Geometry: final body of the model. Coordinates: model frame, mm. Face numbers are marked on the shaded views. Round coordinates to 2 decimals unless told otherwise and drop trailing zeros. Loops run counter-clockwise (first coordinate to the right, second up) from the corner with the lowest first, then second, coordinate; pieces in that order, holes last. Notation, with made-up numbers: M 89,-19.75 L 100,-19.75 A20 ccw 100,12.25 Z; hole C -24.75,4.25 d6. An arc over 180 degrees is marked long. Write each question's results on one line, items separated by ' | '.
```python
from build123d import *

# Parameters (mm, degrees)
F0_R     = 5.5
F1_DEPTH = 13.6
F2_R     = 8.165
F3_DEPTH = 1.82
F4_R     = 5.65
F5_DEPTH = 25
F6_R     = 4.5
F7_DEPTH = 40.421
F8_R     = 1.45
F9_DEPTH = 12


with BuildPart() as f1:
    # F0 (on Top) → F1 (new body)
    with BuildSketch(Plane.XY):
        Circle(F0_R)
    extrude(amount=F1_DEPTH)

    # F2 (on face) → F3 (join)
    with BuildSketch(Plane.XY.offset(13.6)):
        Circle(F2_R)
    extrude(amount=F3_DEPTH)

    # F4 (on face) → F5 (join)
    with BuildSketch(Plane.XY.offset(15.42)):
        Circle(F4_R)
    extrude(amount=F5_DEPTH)

    # F6 (on face) → F7 (cut, through all)
    with BuildSketch(Plane(origin=(0, 0, 0), x_dir=(1, 0, 0), z_dir=(0, 0, -1))):
        Circle(F6_R)
    extrude(amount=-F7_DEPTH, mode=Mode.SUBTRACT)

    # F8 (on Front) → F9 (cut)
    with BuildSketch(Plane.XZ):
        with Locations((0, 25)):
            Circle(F8_R)
        with Locations((0, 5)):
            Circle(F8_R)
    extrude(amount=F9_DEPTH, mode=Mode.SUBTRACT)


solid = f1.part
```
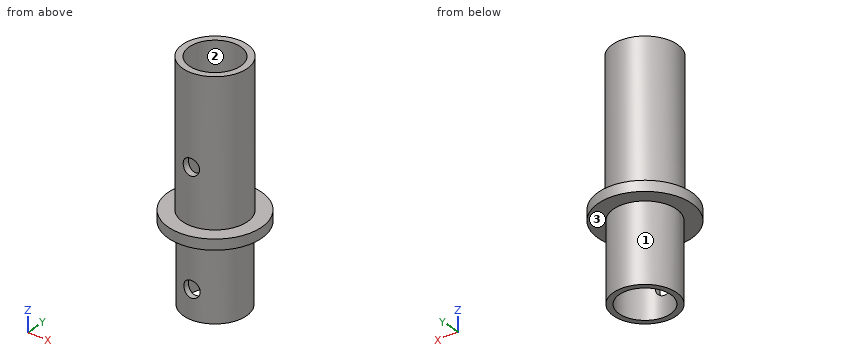
1. Pin query (flat end, axial travel): P1, Ø3, axis at x = -2.5, z = 14.5, coming from the +Y side; P2, Ø4, axis at x = 0, z = 25, coming from the -Y side; P3, Ø1.5, axis at y = -4, z = 11, coming from the +X side. Return the tip coordinate at first contact, or that it passes through.
Answer key:
P1: stops at y = 8.1 | P2: stops at y = -5.65 | P3: stops at x = 4.44
2. Section B-B (x = 0). Output: boundary loops of the cut face in (y, z) (3 decimals), then the cut area to 3 significant figures.
Answer key:
outline: M -8.165,13.6 L -5.5,13.6 L -5.5,6.45 L -4.5,6.45 L -4.5,23.55 L -5.65,23.55 L -5.65,15.42 L -8.165,15.42 Z; M -5.65,26.45 L -4.5,26.45 L -4.5,40.42 L -5.65,40.42 Z; M -5.5,0 L -4.5,0 L -4.5,3.55 L -5.5,3.55 Z; M 4.5,0 L 5.5,0 L 5.5,13.6 L 8.165,13.6 L 8.165,15.42 L 5.65,15.42 L 5.65,40.42 L 4.5,40.42 Z | area: 91.8 mm²
3. Section A-A (y = 0). Output: boundary loops of the cut face in (x, z) (3 decimals).
Answer key:
outline: M -8.165,13.6 L -5.5,13.6 L -5.5,0 L -4.5,0 L -4.5,40.42 L -5.65,40.42 L -5.65,15.42 L -8.165,15.42 Z; M 4.5,0 L 5.5,0 L 5.5,13.6 L 8.165,13.6 L 8.165,15.42 L 5.65,15.42 L 5.65,40.42 L 4.5,40.42 Z
4. Section D-D (x = -3). Output: boundary loops of the cut face in (y, z).
Answer key:
outline: M -7.59,13.6 L -4.61,13.6 L -4.61,0 L -3.35,0 L -3.35,40.42 L -4.79,40.42 L -4.79,15.42 L -7.59,15.42 Z; M 3.35,0 L 4.61,0 L 4.61,13.6 L 7.59,13.6 L 7.59,15.42 L 4.79,15.42 L 4.79,40.42 L 3.35,40.42 Z
5. Ray query, probe 1 along Z at (x, y) = (0, -5.05); probe 2 along Y at (x, z) = (0, 9.5); probe 3 along Y at (x, z) = (0, 21.5). Return the intervals inside material, ascending.
Answer key:
probe 1: z = 0 to 3.55, 6.45 to 23.55, 26.45 to 40.42 | probe 2: y = -5.5 to -4.5, 4.5 to 5.5 | probe 3: y = -5.65 to -4.5, 4.5 to 5.65
6. Section C-C (z = 19.5). Output: boundary loops of the cut face in (x, y).
Answer key:
outline: C 0,0 d11.3; hole C 0,0 d9
7. Draft query along Y for the marked faces 1, 2 and 3. Return one class per face: pulls with the +Y half, pulls with the -Y half, needs draft (parallel to the pull), parting line crosses it, or undercut.
Answer key:
face 1: parting line crosses it | face 2: undercut | face 3: needs draft
